from build123d import *

# Parameters (mm, degrees)
SKETCH_1_R                       = 175
EXTRUDE_1_DEPTH                  = 5
CUT_EXTRUDE_1_DEPTH              = 248.53787589
CUT_EXTRUDE_3_DEPTH              = 248.53787589
M5X0_8_1_D                       = 4.2
HOLE_WIZARD_M4_1_D               = 4.3
FILLET_1_R                       = 10
FILLET_2_R                       = 5
PATTERN_CIRCULAR_1_COUNT         = 3
FILLET_1_OF_PATTERN_CIRCULAR_1_R = 10
FILLET_2_OF_PATTERN_CIRCULAR_1_R = 5
CUT_EXTRUDE_2_DEPTH              = 243.280431899
M4X0_7_1_D                       = 3.3
M4X0_7_2_D                       = 3.3
M4X0_7_3_D                       = 3.3
M4X0_7_4_D                       = 3.3
PATTERN_LINEAR_1_COUNT           = 2
PATTERN_LINEAR_1_PITCH           = 20
SKETCH_30_W                      = 20
SKETCH_30_H                      = 50
CUT_EXTRUDE_4_DEPTH              = 243.280431899
FILLET_3_R                       = 10


with BuildPart() as part:
    # 草圖1 → 填料-伸長1 (new body)
    with BuildSketch(Plane.XY):
        Circle(SKETCH_1_R)
    extrude(amount=EXTRUDE_1_DEPTH)

    # 草圖6 → 除料-伸長1 (cut, through all)
    with BuildSketch(Plane.XY.offset(5)):
        with BuildLine():
            Line((-45, -169.115345253), (-45, -118))
            Line((-45, -118), (45, -118))
            Line((45, -118), (45, -169.115345253))
            ThreePointArc((45, -169.115345253), (0, -175), (-45, -169.115345253))
        make_face()
    cut_extrude_1 = extrude(amount=-CUT_EXTRUDE_1_DEPTH, mode=Mode.SUBTRACT)

    # 草圖12 → 除料-伸長3 (cut, through all)
    with BuildSketch(Plane.XY.offset(5)):
        with BuildLine():
            Line((-117.153745139, 130), (117.153745139, 130))
            ThreePointArc((117.153745139, 130), (0, 175), (-117.153745139, 130))
        make_face()
    extrude(amount=-CUT_EXTRUDE_3_DEPTH, mode=Mode.SUBTRACT)

    # M5x0.8 螺紋孔1 (through all)
    with Locations(Plane.XY.offset(5)):
        with Locations((25, -114), (-25, -114)):
            m5x0_8_1 = Hole(M5X0_8_1_D / 2)

    # M4 餘隙孔1 (through all)
    with Locations(Plane.XY.offset(5)):
        with Locations((10, -51), (-10, -51)):
            hole_wizard_m4_1 = Hole(HOLE_WIZARD_M4_1_D / 2)

    # 圓角1
    fillet_1_edges = [part.edges().sort_by_distance(p)[0] for p in [
        (45, -118, 2.5),
        (-45, -118, 2.5),
    ]]
    fillet(fillet_1_edges, radius=FILLET_1_R)

    # 圓角2
    fillet_2_edges = [part.edges().sort_by_distance(p)[0] for p in [
        (45, -169.115345253, 2.5),
        (-45, -169.115345253, 2.5),
    ]]
    fillet(fillet_2_edges, radius=FILLET_2_R)

    # 環狀複製排列1: 除料-伸長1, M5x0.8 螺紋孔1, M4 餘隙孔1 ×3 about axis
    pattern_circular_1_axis = Axis((0, 0, 0), (0, 0, 1))
    add([cut_extrude_1.rotate(pattern_circular_1_axis, i * 360 / PATTERN_CIRCULAR_1_COUNT) for i in range(1, PATTERN_CIRCULAR_1_COUNT)], mode=Mode.SUBTRACT)
    add([m5x0_8_1.rotate(pattern_circular_1_axis, i * 360 / PATTERN_CIRCULAR_1_COUNT) for i in range(1, PATTERN_CIRCULAR_1_COUNT)], mode=Mode.SUBTRACT)
    add([hole_wizard_m4_1.rotate(pattern_circular_1_axis, i * 360 / PATTERN_CIRCULAR_1_COUNT) for i in range(1, PATTERN_CIRCULAR_1_COUNT)], mode=Mode.SUBTRACT)

    # 圓角1 of 環狀複製排列1
    fillet_1_of_pattern_circular_1_edges = [part.edges().sort_by_distance(p)[0] for p in [
        (79.690997647, 97.97114317, 2.5),
        (124.690997647, 20.02885683, 2.5),
        (-124.690997647, 20.02885683, 2.5),
        (-79.690997647, 97.97114317, 2.5),
    ]]
    fillet(fillet_1_of_pattern_circular_1_edges, radius=FILLET_1_OF_PATTERN_CIRCULAR_1_R)

    # 圓角2 of 環狀複製排列1
    fillet_2_of_pattern_circular_1_edges = [part.edges().sort_by_distance(p)[0] for p in [
        (123.958185159, 123.528815797, 2.5),
        (168.958185159, 45.586529456, 2.5),
        (-168.958185159, 45.586529456, 2.5),
        (-123.958185159, 123.528815797, 2.5),
    ]]
    fillet(fillet_2_of_pattern_circular_1_edges, radius=FILLET_2_OF_PATTERN_CIRCULAR_1_R)

    # 草圖11 → 除料-伸長2 (cut, through all)
    with BuildSketch(Plane.XY.offset(5)):
        Polygon((54.270925304, 0), (27.135462652, 47), (-27.135462652, 47), (-54.270925304, 0), (-27.135462652, -47), (27.135462652, -47), align=None)
    extrude(amount=-CUT_EXTRUDE_2_DEPTH, mode=Mode.SUBTRACT)

    # M4x0.7 螺紋孔1 (through all)
    with Locations(Plane(origin=(0, 0, 0), x_dir=(1, 0, 0), z_dir=(0, 0, -1))):
        with Locations((64, -105), (-40, -105), (40, -105), (-64, -105)):
            Hole(M4X0_7_1_D / 2)

    # M4x0.7 螺紋孔2 (through all)
    with Locations(Plane(origin=(0, 0, 0), x_dir=(-1, 0, 0), z_dir=(0, 0, -1))):
        with Locations((-150, -16), (-150, 8)):
            m4x0_7_2 = Hole(M4X0_7_2_D / 2)

    # 鏡射1: M4x0.7 螺紋孔2 across plane
    add(m4x0_7_2.mirror(Plane(origin=(0, 0, 0), x_dir=(0, 0, 1), z_dir=(1, 0, 0))), mode=Mode.SUBTRACT)

    # M4x0.7 螺紋孔3 (through all)
    with Locations(Plane(origin=(0, 0, 0), x_dir=(-1, 0, 0), z_dir=(0, 0, -1))):
        with Locations((-90, -125), (90, -125), (-66, -125), (66, -125)):
            Hole(M4X0_7_3_D / 2)

    # M4x0.7 螺紋孔4 (through all)
    with Locations(Plane(origin=(0, 0, 0), x_dir=(-1, 0, 0), z_dir=(0, 0, -1))):
        with Locations((-20, 95), (0, 95), (20, 95)):
            m4x0_7_4 = Hole(M4X0_7_4_D / 2)

    # 直線複製排列1: M4x0.7 螺紋孔4 ×2
    with Locations(*[(0, i * PATTERN_LINEAR_1_PITCH, 0) for i in range(1, PATTERN_LINEAR_1_COUNT)]):
        add(m4x0_7_4, mode=Mode.SUBTRACT)

    # 草圖30 → 除料-伸長4 (cut, through all)
    with BuildSketch(Plane(origin=(0, 0, 0), x_dir=(-1, 0, 0), z_dir=(0, 0, -1))):
        with Locations((0, 105)):
            Rectangle(SKETCH_30_W, SKETCH_30_H)
    extrude(amount=-CUT_EXTRUDE_4_DEPTH, mode=Mode.SUBTRACT)

    # 圓角3
    # the kernel refuses this fillet: 10 mm, written as the material it takes off along each edge
    with BuildSketch(Plane(origin=(117.153745139, 130, 14.387351056), x_dir=(-1, 0, 0), z_dir=(0, 0, -1))) as fillet_3_piece_1:
        with BuildLine():
            CenterArc((3.754940422, -10), FILLET_3_R, 90, 34.868690312)
            ThreePointArc((-1.962035679, -1.795355934), (-0.984428411, -0.89395076), (0, 0))
            Line((0, 0), (3.754940422, 0))
        make_face()
    extrude(amount=23.774702112, mode=Mode.SUBTRACT)
    with BuildSketch(Plane(origin=(-117.153745139, 130, 14.387351056), x_dir=(-0.7377488527990645, -0.6750752774273876, 0), z_dir=(0, 0, -1))) as fillet_3_piece_2:
        with BuildLine():
            CenterArc((3.980549785, -9.912355975), FILLET_3_R, 97.591305889, 34.868690312)
            Line((-2.770202989, -2.534867447), (0, 0))
            ThreePointArc((0, 0), (1.329744988, 0.005052135), (2.659489977, 0))
        make_face()
    extrude(amount=23.774702112, mode=Mode.SUBTRACT)


solid = part.part
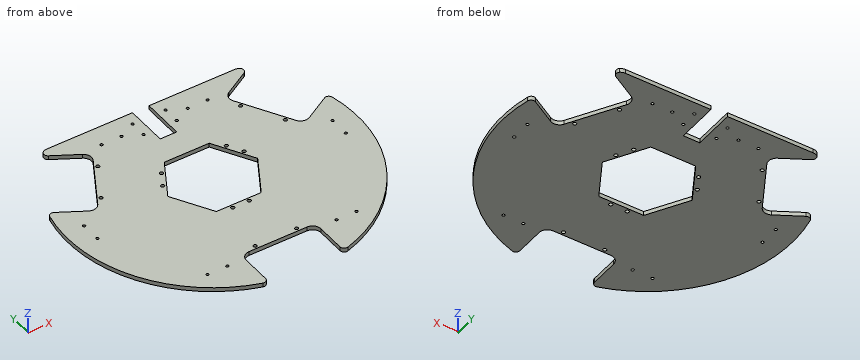
Can you work these out from the model? Positions are in its coordinate system, mm. Coordinates: 2 decimals unless noted, no trailing zeros. Write each loop counter-clockwise with the first axis right and the second up, starting at its lowest first coordinate (ties: lowest second). Pieces come first, ordered by that corner, then holes.
Q1. Please list where these lines run through material, in increasing order: L1, parallel to Y at x = -20, z = 3.45; L2, parallel to X at y = -114.5, z = 1.7; L3, parallel to X at y = 31, z = 4.3.
Results found:
L1: y = -118 to -47, 47 to 93.35, 96.65 to 113.35, 116.65 to 130
L2: x = -132.34 to -27.04, -22.96 to 22.96, 27.04 to 132.34
L3: x = -172.23 to -143.69, -118.36 to -36.37, 36.37 to 118.36, 143.69 to 172.23
Q2. Imagine slicing it at D-D, the plane y = -64. List the corners of the cut face in (x, z) for me.
Results found:
outline: (-162.88, 0) - (162.88, 0) - (162.88, 5) - (-162.88, 5) - close
Q3. Imagine slicing it at B-B, the plane x = 127. List the corners of the cut face in (y, z) for me, plus the area to 3 significant figures.
Results found:
outline: (-120.4, 0) - (23.78, 0) - (23.78, 5) - (-120.4, 5) - close
area: 721 mm2
Q4. Imagine slicing it at A-A, the plane y = -22. List the corners of the cut face in (x, z) for me.
Results found:
outline: (-173.61, 0) - (-41.57, 0) - (-41.57, 5) - (-173.61, 5) - close; (41.57, 0) - (173.61, 0) - (173.61, 5) - (41.57, 5) - close
Q5. Imagine slicing it at C-C, the plane z = 3.7. Count the separate pieces of the cut face and the enclosed holes in it, plus the area to 3 significant figures.
Results found:
separate pieces: 1
enclosed holes: 29
area: 65,200 mm2
Q6. For P1, Ø4, axis at x = 90, y = -125, coming from the +Z side; P2, Ø2, axis at x = -45.5, z = 0.5, coming from the -Y side; P3, Ø2.5, axis at y = 109.5, z = 2, coming from the -X side; P4, Ø1.5, axis at x = 4, z = 3.5, coming from the +Y side, each with a flat end and sliding along its axis, tell me the tip position at first contact or that it passes through.
Results found:
P1: stops at z = 5
P2: stops at y = -166.05
P3: stops at x = -101.82
P4: stops at y = 80
